from build123d import *

# Parameters (mm, degrees)
F1_DEPTH = 700
F2_W     = 924.519062
F2_H     = 457.303435
F3_DEPTH = 392
F4_W     = 1921.999932
F4_H     = 721.999932
F5_DEPTH = 152


with BuildPart() as f1:
    # F0 (on Top) → F1 (new body)
    with BuildSketch(Plane.XY):
        Polygon((-500, -250), (0, -250), (1500, -250), (1500, 0), (1500, 550), (-500, 550), align=None)
    extrude(amount=F1_DEPTH)

    # F2 (on face) → F3 (cut)
    with BuildSketch(Plane.XZ.offset(250)):
        with Locations((462.259531, 228.651717)):
            Rectangle(F2_W, F2_H)
    extrude(amount=-F3_DEPTH, mode=Mode.SUBTRACT)

    # F4 (on face) → F5 (cut)
    with BuildSketch(Plane.XY.offset(700)):
        with Locations((500, 150)):
            Rectangle(F4_W, F4_H)
    extrude(amount=-F5_DEPTH, mode=Mode.SUBTRACT)


solid = f1.part
Here's how the part is built. I have some questions about the finished solid (model axes, mm). A direction names the side the tool comes from. Coordinates: 2 decimals unless noted, no trailing zeros. Write each loop counter-clockwise with the first axis right and the second up, starting at its lowest first coordinate (ties: lowest second). Pieces come first, ordered by that corner, then holes.
Item 1: I want a section at B-B on z = 409. Write out the boundary of the cut face in (x, y).
Item 2: On a 3-axis mill with a long thin cutter (end or side, diameter ignored), from which of +Z, -Z, +X, -X, +Y, -Y can I reach the whole of each face in a straight line? I mean faces 1 (the flat face through (456, -57, 457.303)), 2 (the flat face through (487, -211, 625)), 3 (the flat face through (486, -250, 501)). Say none if no direction works.
Item 3: Will these pins go through, and if not, where does the flat tip stop? pin 1 (6 mm diameter, centred on x = 1066.5, y = 255, fed in from +Z); pin 2 (10 mm diameter, centred on x = 585.5, z = 251.5, fed in from -Y).
Item 4: If we mould it in two halves opening along Y, with no side actions, what happens to faces 4 (the flat face through (514, 550, 345)), 5 (the flat face through (924.519, -57, 225)), 6 (the flat face through (487, 155, 548)), 7 (the flat face through (456, 142, 232))? For each: +Y half, -Y half, draft (parallel to the pull), parting line (faces both ways), or undercut.
Item 5: I want a section at D-D on y = 118.5. Write out the boundary of the cut face in (x, z), and give its area (3 significant figures).
Item 6: I want a section at A-A on y = 282.5. Write out the boundary of the cut face in (x, z), and give its area (3 significant figures).
Item 7: I want a section at C-C on x = 270. Write out the boundary of the cut face in (y, z).
Item 8: If I drill on line 1 (Y direction, x = 49, z = 594); line 2 (X direction, y = -106, z = 170.5); line 3 (X direction, y = -53.5, z = 551), over which ranges is the centre line in solid material (lowest first)?
Findings below:
1. outline: (-500, -250) - (0, -250) - (0, 142) - (924.52, 142) - (924.52, -250) - (1500, -250) - (1500, 550) - (-500, 550) - close
2. face 1: -Z, -Y
2. face 2: +Z
2. face 3: +Z, -Z, +X, -X, -Y
3. pin 1: stops at z = 548
3. pin 2: stops at y = 142
4. face 4: +Y half
4. face 5: draft
4. face 6: undercut
4. face 7: -Y half
5. outline: (-500, 0) - (0, 0) - (0, 457.3) - (924.52, 457.3) - (924.52, 0) - (1500, 0) - (1500, 700) - (1461, 700) - (1461, 548) - (-461, 548) - (-461, 700) - (-500, 700) - close
5. area: 685,000 mm2
6. outline: (-500, 0) - (1500, 0) - (1500, 700) - (1461, 700) - (1461, 548) - (-461, 548) - (-461, 700) - (-500, 700) - close
6. area: 1,110,000 mm2
7. outline: (-250, 457.3) - (142, 457.3) - (142, 0) - (550, 0) - (550, 700) - (511, 700) - (511, 548) - (-211, 548) - (-211, 700) - (-250, 700) - close
8. line 1: y = -250 to -211, 511 to 550
8. line 2: x = -500 to 0, 924.52 to 1500
8. line 3: x = -500 to -461, 1461 to 1500
